Part print with two shaded views. Sizes in mm from the minimum x, y, z corner. Coordinates: 2 decimals unless noted, no trailing zeros. Loops run counter-clockwise (first coordinate to the right, second up) from the corner with the lowest first, then second, coordinate; pieces in that order, holes last.
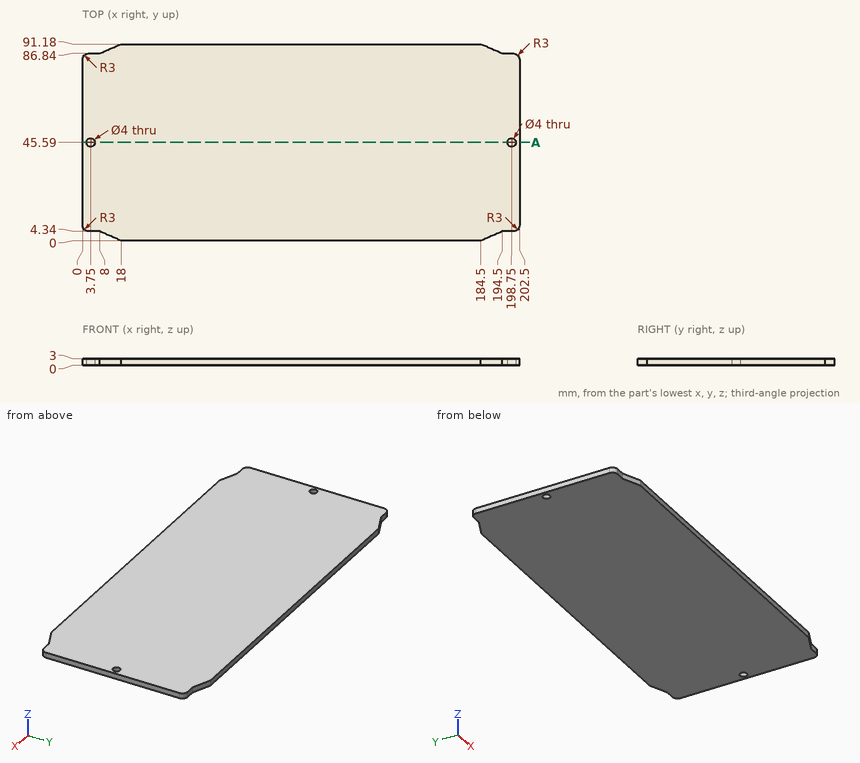
Q1. Drill centre lines: line 1 (Y direction, x = 198.75, z = 0.6); line 2 (X direction, y = 84, z = 1.95); line 3 (Y direction, x = 9, z = 0.6). Where is each one in solid material? Low to high.
Answers:
line 1: y = 4.34 to 43.59, 47.59 to 86.84
line 2: x = 0 to 202.5
line 3: y = 3.91 to 87.27
Q2. Slice it at A-A (y = 45.59). List the corners of the cut face in (x, z).
Answers:
outline: (0, 0) - (1.75, 0) - (1.75, 3) - (0, 3) - close; (5.75, 0) - (196.75, 0) - (196.75, 3) - (5.75, 3) - close; (200.75, 0) - (202.5, 0) - (202.5, 3) - (200.75, 3) - close
Q3. Flat gauge pins, fed straight in: P1, Ø0.9, axis at x = 5, z = 1.5, coming from the -Y side; P2, Ø3, axis at x = 3.75, y = 45.59, coming from the +Z side. Where does each tip first touch, or does it go through?
Answers:
P1: stops at y = 4.34
P2: passes through
